Geometry check sheet. Reference: the model listing, model coordinates, mm. Coordinates: 2 decimals unless noted, no trailing zeros. Write each loop counter-clockwise with the first axis right and the second up, starting at its lowest first coordinate (ties: lowest second). Pieces come first, ordered by that corner, then holes. Notation, with made-up numbers: (63, 68) -> (102, 68) arc R35 cw to (102, 100) -> close; hole circle Ø1 at (12.5, 24.5). An arc over 180 degrees is marked (long way). Answer in a Markdown table with one row per item. Add a question column.
1. Scan lines: L1, parallel to X at y = 2.5, z = 3.55; L2, parallel to Y at x = 13.3, z = 1.95; L3, parallel to Y at x = 22.25, z = 1.75. Record each from-to range of solid material in increasing order. Write a range as from..to.
2. Depth check by flat-ended pin: P1, Ø3, axis at y = 28, z = -0.5, coming from the +X side; P2, Ø2, axis at x = 2.8, y = 2.5, coming from the -Z side. Enter the tip coordinate at first touch or a pass-through.
3. Cross-section at B-B on y = 39. Record the cut outline in (x, z), and give its area (3 significant figures).
4. Cross-section at A-A on x = 13.3. Record the cut outline in (y, z).
5. Cross-section at D-D on y = 8. Record the cut outline in (x, z).
6. Cross-section at C-C on y = 2.5. Record the cut outline in (x, z), and give its area (3 significant figures).
Autodesk Inventor part; units mm, degrees
ref_plane "YZ Plane" through (0, 0, 0) normal (1, 0, 0) x (0, 1, 0)
ref_plane "XZ Plane" through (0, 0, 0) normal (0, 1, 0) x (-1, 0, 0)
ref_plane "XY Plane" through (0, 0, 0) normal (0, 0, 1) x (1, 0, 0)
sketch "Sketch1" plane through (0, 0, 0) normal (0, 0, 1) x (1, 0, 0)
  line L0 (0, 0) -> (25, 0)
  line L1 (25, 0) -> (25, 50)
  line L2 (25, 50) -> (0, 50)
  line L3 (0, 50) -> (0, 0)
  dimension "d0" = 50
  dimension "d1" = 25
extrude "Extrusion1" add sketch "Sketch1" along normal blind 5
sketch "Sketch7" plane through (0, 0, 0) normal (0, 0, -1) x (-1, 0, 0)
  line L0 (0, 0) -> (-25, 0)
  line L1 (0, 50) -> (0, 0)
  line L2 (-25, 50) -> (0, 50)
  line L3 (-25, 0) -> (-25, 50)
  line L4 (-26.9321, 31.3954) -> (-26.9317, 31.395)
  line L5 (-6.036, 52.1675) -> (-6.0379, 52.1694)
  line L6 (-6.0392, 52.1707) -> (-6.0403, 52.1719)
  line L7 (-25, 50) -> (-17.5538, 50)
  line L8 (-9.8347, 48.3993) -> (-9.8243, 48.3993)
  line L9 (-25, 50) -> (-25, 43.2194)
  line L10 (-25, 33.3181) -> (-25, 33.3148)
  line L11 (-25, 50) -> (-25, 0)
  line L12 (-25, 0) -> (0, 0)
  line L13 (0, 0) -> (0, 50)
  line L14 (-4.3266, 37.6341) -> (0, 42.0051)
  line L15 (-7.4462, 50) -> (-12.072, 45.3663)
  line L16 (-12.072, 45.3663) -> (-4.3266, 37.6341)
  line L17 (-12.072, 45.3663) -> (-4.3266, 37.6341)
  point P0 (0, 33.3148)
  point P1 (0, 45.3321)
  point P2 (0, 37.6341)
  point P3 (-16.7135, 50)
  point P4 (0, 42.0051)
  dimension "d59" = 16.7135
  dimension "d60" = 7.4462
extrude "Extrusion3" add sketch "Sketch7" along normal blind 2 from surface at 0 contours L14 L16 L15 L2 L1
sketch "Sketch11" plane through (0, 0, 0) normal (0, 0, -1) x (-1, 0, 0)
  circle A0 centre (-13.3, 39.8488) radius 1.651
  line L0 (-25, 50) -> (-7.4462, 50)
  line L1 (-25, 0) -> (-25, 50)
  point P0 (0, 0)
  dimension "d61" = 3.302
  dimension "d62" = 10.1512
  dimension "d63" = 11.7
hole "Hole5" at (13.3, 39.8488, 0) direction (0, 0, 1) diameter 3.302 end through all
sketch "Sketch12" plane through (0, 0, 0) normal (0, 0, -1) x (-1, 0, 0)
  circle A0 centre (-22.8048, 22.5) radius 0.847
  line L0 (0, 0) -> (-25, 0)
  line L1 (-25, 0) -> (-25, 50)
  circle A1 centre (-22.8048, 2.5) radius 0.847
  circle A2 centre (-2.8048, 22.5) radius 0.847
  line L2 (0, 42.0051) -> (0, 0)
  circle A3 centre (-2.8048, 2.5) radius 0.847
  dimension "d71" = 1.694
  dimension "d72" = 22.5
  dimension "d73" = 2.1952
  dimension "d74" = 1.694
  dimension "d75" = 20
  dimension "d76" = 2.8048
  dimension "d77" = 1.694
  dimension "d78" = 1.694
hole "Hole8" at (22.8048, 22.5, 0) at (22.8048, 2.5, 0) at (2.8048, 22.5, 0) at (2.8048, 2.5, 0) direction (0, 0, 1) diameter 1.6942 end through all
properties part number "mirror translation stage adapter v2"
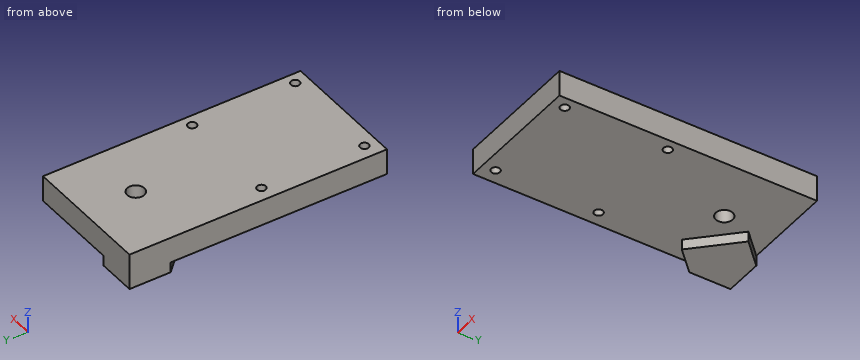
Results found:
| question | item | result |
|---|---|---|
| 1 | L1 | x = 0..1.96, 3.65..21.96, 23.65..25 |
| 1 | L2 | y = 0..38.2, 41.5..50 |
| 1 | L3 | y = 0..1.86, 3.14..21.86, 23.14..50 |
| 2 | P1 | stops at x = 25 |
| 2 | P2 | stops at z = 0 |
| 3 | outline | (0, 0) -> (2.97, 0) -> (2.97, -2) -> (5.69, -2) -> (5.69, 0) -> (11.88, 0) -> (11.88, 5) -> (0, 5) -> close; (14.72, 0) -> (25, 0) -> (25, 5) -> (14.72, 5) -> close |
| 3 | area | 116 mm^2 |
| 4 | outline | (0, 0) -> (38.2, 0) -> (38.2, 5) -> (0, 5) -> close; (41.5, 0) -> (50, 0) -> (50, 5) -> (41.5, 5) -> close |
| 5 | outline | (0, 0) -> (25, 0) -> (25, 5) -> (0, 5) -> close |
| 6 | outline | (0, 0) -> (1.96, 0) -> (1.96, 5) -> (0, 5) -> close; (3.65, 0) -> (21.96, 0) -> (21.96, 5) -> (3.65, 5) -> close; (23.65, 0) -> (25, 0) -> (25, 5) -> (23.65, 5) -> close |
| 6 | area | 108 mm^2 |
